from build123d import *

# Parameters (mm, degrees)
BOSS_EXTRU_1_DEPTH      = 3
ESQUISSE2_R             = 10
BOSS_EXTRU_2_DEPTH      = 7
BOSS_EXTRU_3_DEPTH      = 5
ESQUISSE4_W             = 12
ESQUISSE4_H             = 28
ENL_V_MAT_EXTRU_1_DEPTH = 5


# Read off the part's stored shape, not the designer's step: Boss.-Extru.1
with BuildPart() as part:
    # Boss.-Extru.1 outline → Boss.-Extru.1 (new body)
    with BuildSketch(Plane.XY):
        with BuildLine():
            ThreePointArc((-25.25, -4.5), (-20.710155108, -15.460155108), (-9.75, -20))
            Line((-9.75, -20), (9.75, -20))
            ThreePointArc((9.75, -20), (20.710155108, -15.460155108), (25.25, -4.5))
            Line((25.25, -4.5), (25.25, -4))
            Line((25.25, -4), (30.83484861, -4))
            ThreePointArc((30.83484861, -4), (50, 0), (30.83484861, 4))
            Line((30.83484861, 4), (25.25, 4))
            Line((25.25, 4), (25.25, 21))
            Line((25.25, 21), (28, 21))
            Line((28, 21), (28, 11))
            Line((28, 11), (40, 11))
            Line((40, 11), (40, 39))
            Line((40, 39), (28, 39))
            Line((28, 39), (28, 29))
            Line((28, 29), (25.25, 29))
            Line((25.25, 29), (25.25, 35))
            ThreePointArc((25.25, 35), (20.710155108, 45.960155108), (9.75, 50.5))
            Line((9.75, 50.5), (4, 50.5))
            Line((4, 50.5), (4, 52.282032303))
            Line((4, 52.282032303), (21.172408726, 52.282032303))
            Line((21.172408726, 52.282032303), (26.332088428, 42.535970645))
            Line((26.332088428, 42.535970645), (36.937543424, 48.15062329))
            Line((36.937543424, 48.15062329), (23.836687252, 72.896684948))
            Line((23.836687252, 72.896684948), (13.231232256, 67.282032303))
            Line((13.231232256, 67.282032303), (17.995938138, 58.282032303))
            Line((17.995938138, 58.282032303), (4, 58.282032303))
            Line((4, 58.282032303), (4, 60.116880913))
            ThreePointArc((4, 60.116880913), (0, 79.282032303), (-4, 60.116880913))
            Line((-4, 60.116880913), (-4, 58.282032303))
            Line((-4, 58.282032303), (-17.995938138, 58.282032303))
            Line((-17.995938138, 58.282032303), (-13.231232256, 67.282032303))
            Line((-13.231232256, 67.282032303), (-23.836687252, 72.896684948))
            Line((-23.836687252, 72.896684948), (-36.937543424, 48.15062329))
            Line((-36.937543424, 48.15062329), (-26.332088428, 42.535970645))
            Line((-26.332088428, 42.535970645), (-21.172408726, 52.282032303))
            Line((-21.172408726, 52.282032303), (-4, 52.282032303))
            Line((-4, 52.282032303), (-4, 50.5))
            Line((-4, 50.5), (-9.75, 50.5))
            ThreePointArc((-9.75, 50.5), (-20.710155108, 45.960155108), (-25.25, 35))
            Line((-25.25, 35), (-25.25, 29))
            Line((-25.25, 29), (-28, 29))
            Line((-28, 29), (-28, 39))
            Line((-28, 39), (-40, 39))
            Line((-40, 39), (-40, 11))
            Line((-40, 11), (-28, 11))
            Line((-28, 11), (-28, 21))
            Line((-28, 21), (-25.25, 21))
            Line((-25.25, 21), (-25.25, 4))
            Line((-25.25, 4), (-30.83484861, 4))
            ThreePointArc((-30.83484861, 4), (-50, 0), (-30.83484861, -4))
            Line((-30.83484861, -4), (-25.25, -4))
            Line((-25.25, -4), (-25.25, -4.5))
        make_face()
    extrude(amount=BOSS_EXTRU_1_DEPTH)

    # Esquisse2 → Boss.-Extru.2 (add)
    with BuildSketch(Plane.XY.offset(3)):
        with Locations(Location((-40, 0, 0), (0, 0, 336.421821522))):
            Circle(ESQUISSE2_R)
        with Locations(Location((40, 0, 0), (0, 0, 156.421821522))):
            Circle(ESQUISSE2_R)
        with Locations(Location((0, 69.282032303, 0), (0, 0, 246.421821522))):
            Circle(ESQUISSE2_R)
    extrude(amount=BOSS_EXTRU_2_DEPTH)

    # Esquisse3 → Boss.-Extru.3 (add)
    with BuildSketch(Plane.XY.offset(3)):
        Polygon((23.836687252, 72.896684948), (36.937543424, 48.15062329), (26.332088428, 42.535970645), (21.172408726, 52.282032303), (-21.172408726, 52.282032303), (-26.332088428, 42.535970645), (-36.937543424, 48.15062329), (-23.836687252, 72.896684948), (-13.231232256, 67.282032303), (-17.995938138, 58.282032303), (17.995938138, 58.282032303), (13.231232256, 67.282032303), align=None)
        Polygon((28, 39), (40, 39), (40, 11), (28, 11), (28, 21), (-28, 21), (-28, 11), (-40, 11), (-40, 39), (-28, 39), (-28, 29), (28, 29), align=None)
    extrude(amount=BOSS_EXTRU_3_DEPTH)

    # Esquisse4 → Enlèv. mat.-Extru.1 (cut)
    with BuildSketch(Plane(origin=(0, 0, 0), x_dir=(-1, 0, 0), z_dir=(0, 0, -1))):
        with Locations((-34, 25)):
            Rectangle(ESQUISSE4_W, ESQUISSE4_H)
        Polygon((-36.937543424, 48.15062329), (-26.332088428, 42.535970645), (-13.231232256, 67.282032303), (-23.836687252, 72.896684948), align=None)
        Polygon((13.231232256, 67.282032303), (23.836687252, 72.896684948), (36.937543424, 48.15062329), (26.332088428, 42.535970645), align=None)
        with Locations((34, 25)):
            Rectangle(ESQUISSE4_W, ESQUISSE4_H)
    extrude(amount=-ENL_V_MAT_EXTRU_1_DEPTH, mode=Mode.SUBTRACT)


solid = part.part
Can you work these out from the model? Positions are in its coordinate system, mm. A direction names the side the tool comes from. Coordinates: 2 decimals unless noted, no trailing zeros. Loops run counter-clockwise (first coordinate to the right, second up) from the corner with the lowest first, then second, coordinate; pieces in that order, holes last. Notation, with made-up numbers: M 29.5,47 L 86.5,47 A31 cw 86.5,75 Z; hole C -24,-20 d2. An arc over 180 degrees is marked long. Return JSON: item names as keys, results as strings. Group by question number.
Item 1: Imagine slicing it at C-C (y = 0). Please give me the cut outline in (x, z).
Item 2: I'm going to push flat-ended pins straight in: pin 1 Ø0.9 at (x, z) = (34, 6) entering from -Y; pin 2 Ø0.9 at (y, z) = (14.5, 6.5) entering from +X; pin 3 Ø5 at (x, z) = (-38, 2) entering from +Y. Where does each tip first touch, or does it pass through?
Item 3: Thinking about a two-plate mould opening in Y: for faces 6 (the flat face through (25, 58, 5)), 7 (the flat face through (-28, 34, 6)), 8 (the flat face through (30.295, 60.697, 6.479)), which applies, released by +Y, released by -Y, zero draft, split by the parting line, or undercut?
Item 4: Imagine slicing it at B-B (x = 0). Please give me the cut outline in (y, z), and give its area (3 significant figures).
Item 5: Imagine slicing it at A-A (z = 6.75). Please give me the cut outline in (x, y), and give its area (3 significant figures).
Item 6: If I drill on L1, parallel to X at y = 36, z = 5.5; L2, parallel to Y at x = 16.5, z = 4; L3, parallel to Z at x = -17, y = 39, over which ranges is the centre line in solid material (lowest first)? Write a range as from..to.
Item 7: Imagine slicing it at D-D (y = 65). Please give me the cut outline in (x, z).
Item 8: On a 3-axis mill with a long thin cutter (end or side, diameter ignored), from which of +Z, -Z, +X, -X, +Y, -Y can I reach the whole of each face in a straight line? I mean faces 1 (the flat face through (-7, 50.5, 1)), 2 (the flat face through (0, 29, 5)), 3 (the flat face through (25.25, 12, 1)), 4 (the flat face through (28, -4, 1)), 5 (the flat face through (28, 25, 2)). Say none if no direction works.
Verdict:
{
 "1": {"outline": "M -50,0 L 50,0 L 50,10 L 30,10 L 30,3 L -30,3 L -30,10 L -50,10 Z"},
 "2": {"pin 1": "stops at y = -8.32", "pin 2": "stops at x = 40", "pin 3": "stops at y = 10"},
 "3": {"face 6": "zero draft", "face 7": "undercut", "face 8": "released by +Y"},
 "4": {"outline": "M -20,0 L 79.28,0 L 79.28,10 L 59.28,10 L 59.28,3 L 58.28,3 L 58.28,8 L 52.28,8 L 52.28,3 L 29,3 L 29,8 L 21,8 L 21,3 L -20,3 Z", "area": "508 mm^2"},
 "5": {"outline": "C -40,0 d20; M -40,11 L -28,11 L -28,21 L 28,21 L 28,11 L 40,11 L 40,39 L 28,39 L 28,29 L -28,29 L -28,39 L -40,39 Z; M -36.94,48.15 L -26.33,42.54 L -21.17,52.28 L 21.17,52.28 L 26.33,42.54 L 36.94,48.15 L 23.84,72.9 L 13.23,67.28 L 18,58.28 L -18,58.28 L -13.23,67.28 L -23.84,72.9 Z; C 0,69.28 d20; C 40,0 d20", "area": "2,970 mm^2"},
 "6": {"L1": "x = -40..-28, 28..40", "L2": "y = 21..29, 52.28..58.28", "L3": "z = 0..3"},
 "7": {"outline": "M -28.02,5 L -14.44,5 L -14.44,8 L -28.02,8 Z; M -9.04,0 L 9.04,0 L 9.04,10 L -9.04,10 Z; M 14.44,5 L 28.02,5 L 28.02,8 L 14.44,8 Z"},
 "8": {"face 1": "+Z, -Z, -X", "face 2": "+Z", "face 3": "+Z, -Z", "face 4": "+Z, -Z, -Y", "face 5": "-Z, +X, +Y"}
}
